Input: part model. Units: mm. Frame: model coordinates. A direction names the side the tool comes from. Give positions to 0.01 mm unless a question says otherwise; leave off trailing zeros. Loops run counter-clockwise (first coordinate to the right, second up) from the corner with the lowest first, then second, coordinate; pieces in that order, holes last. Notation, with made-up numbers: (1.5, 19.25) -> (53.5, 19.25) arc R25 ccw to (53.5, 37.25) -> close; hole circle Ø11 at (-33.75, 0). An arc over 180 degrees is marked (long way). Answer in a Markdown table with one row per item. Add a question column.
```python
from build123d import *

# Parameters (mm, degrees)
CROQUIS1_W              = 150
CROQUIS1_H              = 80
CROQUIS1_W_2            = 2.3
CROQUIS1_H_2            = 9.5
SALIENTE_EXTRUIR1_DEPTH = 3


with BuildPart() as part:
    # Croquis1 → Saliente-Extruir1 (new body)
    with BuildSketch(Plane(origin=(0, 0, 0), x_dir=(1, 0, 0), z_dir=(0, 1, 0))):
        Rectangle(CROQUIS1_W, CROQUIS1_H)
        with Locations((56.85, 20)):
            Rectangle(CROQUIS1_W_2, CROQUIS1_H_2, mode=Mode.SUBTRACT)
        with Locations((56.85, 0)):
            Rectangle(CROQUIS1_W_2, CROQUIS1_H_2, mode=Mode.SUBTRACT)
        with Locations((56.85, -20)):
            Rectangle(CROQUIS1_W_2, CROQUIS1_H_2, mode=Mode.SUBTRACT)
        with Locations((-56.85, 20)):
            Rectangle(CROQUIS1_W_2, CROQUIS1_H_2, mode=Mode.SUBTRACT)
        with Locations((-56.85, -20)):
            Rectangle(CROQUIS1_W_2, CROQUIS1_H_2, mode=Mode.SUBTRACT)
        with Locations((-56.85, 0)):
            Rectangle(CROQUIS1_W_2, CROQUIS1_H_2, mode=Mode.SUBTRACT)
    extrude(amount=SALIENTE_EXTRUIR1_DEPTH)


solid = part.part
```
1) Material intervals for line 1 along X through (y, z) = (0.1, -1), sorted ascending.
2) Reachability of faces 5 (the face through (-58, 1, 0)), 6 (the face through (-1, 0, -1)) from +Z, -Z, +X, -X, +Y, -Y: full face, straight path, thin tool, end or side. Return the list, or none.
3) Section A-A on z = -2. Output: boundary loops of the cut face in (x, y).
4) Pull-direction query (X, two-part tool) for faces 1 (the face through (58, 1, 20)), 2 (the face through (-75, 1, 1)), 3 (the face through (-1, 1, 40)), 4 (the face through (-55.7, 1, 20)); classes: +X half, -X half, draft (parallel to the pull), parting line (faces both ways), or undercut.
Working result:
| question | item | result |
|---|---|---|
| 1 | line 1 | x = -75 to -58, -55.7 to 55.7, 58 to 75 |
| 2 | face 5 | +Y, -Y |
| 2 | face 6 | +Z, -Z, +X, -X, -Y |
| 3 | outline | (-75, 0) -> (-58, 0) -> (-58, 3) -> (-75, 3) -> close; (-55.7, 0) -> (55.7, 0) -> (55.7, 3) -> (-55.7, 3) -> close; (58, 0) -> (75, 0) -> (75, 3) -> (58, 3) -> close |
| 4 | face 1 | undercut |
| 4 | face 2 | -X half |
| 4 | face 3 | draft |
| 4 | face 4 | undercut |
